Verification items for the finished model (mm, model axes). A direction names the side the tool comes from. Coordinates: 2 decimals unless noted, no trailing zeros. Loops run counter-clockwise (first coordinate to the right, second up) from the corner with the lowest first, then second, coordinate; pieces in that order, holes last. Notation, with made-up numbers: (50, 41) - (59, 41) arc R7 ccw to (59, 50) - close; hole circle Ø5 at (70, 80). An arc over 180 degrees is marked (long way). One line per item, written item: value. Start each with the question number.
(1) Gauge pin test, flat ends, axial feed: P1, Ø3, axis at x = -3, y = -25.5, coming from the +Z side; P2, Ø2.5, axis at x = -22.01, y = -47, coming from the +Z side. Record the tip position at first contact, or that the pin passes through.
(2) Section check A-A (z = 9.5). Count the separate pieces of the cut face and the enclosed holes in it, plus the area to 3 significant figures.
(3) Section check B-B (y = -38). Record the boundary of the cut face in (x, z).
(4) Section check D-D (z = 3.75). Record the boundary of the cut face in (x, y).
(5) Thickness scan on probe 1 along Y at (x, z) = (-22, 4.5); probe 2 along Y at (x, z) = (6, 4); probe 3 along Z at (x, y) = (-0.5, -23). Record the ranges inside material, lowest first. Write a range as [from, to].
(6) Draft check along Z on faces 3 (the face through (0, 1, 0)), 4 (the face through (0, 29, 2)), 5 (the face through (0, 50, 6)), 6 (the face through (0, 1, 8)). Enter one of: +Z half, -Z half, draft (parallel to the pull), parting line (faces both ways), or undercut.
(7) Section check C-C (x = -7). Record the boundary of the cut face in (y, z).
(8) Set-up check for faces 1 (the face through (-24.15, -49.1, 7.4)), 2 (the face through (0, 29, 5)): record each of +Z, -Z, +X, -X, +Y, -Y from which the full face is reachable in a straight line by a thin tool's end or side.
```python
from build123d import *

# Parameters (mm, degrees)
SKETCH1_R           = 2
BOSS_EXTRUDE1_DEPTH = 15
CUT_EXTRUDE1_DEPTH  = 105.165020701
CUT_EXTRUDE2_START  = -10
CUT_EXTRUDE2_DEPTH  = 22
CUT_EXTRUDE3_START  = -68
CUT_EXTRUDE3_DEPTH  = 22


with BuildPart() as part:
    # Sketch1 → Boss-Extrude1 (new body)
    with BuildSketch(Plane.XY):
        with BuildLine():
            Line((-22.007029764, -50.000223574), (21.992970236, -50.000223574))
            ThreePointArc((21.992970236, -50.000223574), (24.114290579, -49.121543918), (24.992970236, -47.000223574))
            Line((24.992970236, -47.000223574), (24.992970236, 46.999776426))
            ThreePointArc((24.992970236, 46.999776426), (24.114290579, 49.12109677), (21.992970236, 49.999776426))
            Line((21.992970236, 49.999776426), (-22.007029764, 49.999776426))
            ThreePointArc((-22.007029764, 49.999776426), (-24.128350108, 49.12109677), (-25.007029764, 46.999776426))
            Line((-25.007029764, 46.999776426), (-25.007029764, -47.000223574))
            ThreePointArc((-25.007029764, -47.000223574), (-24.128350108, -49.121543918), (-22.007029764, -50.000223574))
        make_face()
        with Locations((-22.007029764, 46.999776426)):
            Circle(SKETCH1_R, mode=Mode.SUBTRACT)
        with Locations((21.992970236, 46.999776426)):
            Circle(SKETCH1_R, mode=Mode.SUBTRACT)
        with Locations((21.992970236, -47.000223574)):
            Circle(SKETCH1_R, mode=Mode.SUBTRACT)
        with Locations((-22.007029764, -47.000223574)):
            Circle(SKETCH1_R, mode=Mode.SUBTRACT)
    extrude(amount=BOSS_EXTRUDE1_DEPTH)

    # Sketch2 → Cut-Extrude1 (cut, through all)
    with BuildSketch(Plane(origin=(0, 49.999776426, 0), x_dir=(1, 0, 0), z_dir=(0, 1, 0))):
        with BuildLine():
            ThreePointArc((12.68857754, -15), (0, -8), (-12.68857754, -15))
            Line((-12.68857754, -15), (12.68857754, -15))
        make_face()
    extrude(amount=-CUT_EXTRUDE1_DEPTH, mode=Mode.SUBTRACT)

    # Sketch2<4> → Cut-Extrude2 (cut)
    with BuildSketch(Plane(origin=(0, 49.999776426, 0), x_dir=(1, 0, 0), z_dir=(0, 1, 0)).offset(CUT_EXTRUDE2_START)):
        with BuildLine():
            ThreePointArc((19.416487839, -15), (0, -2), (-19.416487839, -15))
            Line((-19.416487839, -15), (-16.124515497, -15))
            ThreePointArc((-16.124515497, -15), (0, -5), (16.124515497, -15))
            Line((16.124515497, -15), (19.416487839, -15))
        make_face()
    extrude(amount=-CUT_EXTRUDE2_DEPTH, mode=Mode.SUBTRACT)

    # Sketch2<5> → Cut-Extrude3 (cut)
    with BuildSketch(Plane(origin=(0, 49.999776426, 0), x_dir=(1, 0, 0), z_dir=(0, 1, 0)).offset(CUT_EXTRUDE3_START)):
        with BuildLine():
            ThreePointArc((19.416487839, -15), (0, -2), (-19.416487839, -15))
            Line((-19.416487839, -15), (-16.124515497, -15))
            ThreePointArc((-16.124515497, -15), (0, -5), (16.124515497, -15))
            Line((16.124515497, -15), (19.416487839, -15))
        make_face()
    extrude(amount=-CUT_EXTRUDE3_DEPTH, mode=Mode.SUBTRACT)


solid = part.part
```
Responses:
1. P1: stops at z = 8.69
1. P2: passes through
2. separate pieces: 2
2. enclosed holes: 8
2. area: 3,270 mm²
3. outline: (-25.01, 0) - (24.99, 0) - (24.99, 15) - (19.42, 15) arc R21 cw to (-19.42, 15) - (-25.01, 15) - close; (-16.12, 15) arc R18 ccw to (16.12, 15) - (12.69, 15) arc R15 cw to (-12.69, 15) - close
4. outline: (-25.01, -47) arc R3 ccw to (-22.01, -50) - (21.99, -50) arc R3 ccw to (24.99, -47) - (24.99, 47) arc R3 ccw to (21.99, 50) - (-22.01, 50) arc R3 ccw to (-25.01, 47) - close; hole circle Ø4 at (-22.01, -47); hole circle Ø4 at (-22.01, 47); hole (-8.39, -40) - (8.39, -40) - (8.39, -18) - (-8.39, -18) - close; hole (-8.39, 18) - (8.39, 18) - (8.39, 40) - (-8.39, 40) - close; hole circle Ø4 at (21.99, -47); hole circle Ø4 at (21.99, 47)
5. probe 1: y = [-50, -49], [-45, 45], [49, 50]
5. probe 2: y = [-50, -40], [-18, 18], [40, 50]
5. probe 3: z = [0, 2.01], [5.01, 8.01]
6. face 3: -Z half
6. face 4: undercut
6. face 5: draft
6. face 6: +Z half
7. outline: (-50, 0) - (50, 0) - (50, 9.73) - (-50, 9.73) - close; hole (-40, 3.2) - (-18, 3.2) - (-18, 6.42) - (-40, 6.42) - close; hole (18, 3.2) - (40, 3.2) - (40, 6.42) - (18, 6.42) - close
8. face 1: +Z, -Z, -X, -Y
8. face 2: none
